Check sheet for the modelled part. Datum: model origin and axes. Units: mm. Round coordinates to 2 decimals unless told otherwise and drop trailing zeros. Loops run counter-clockwise (first coordinate to the right, second up) from the corner with the lowest first, then second, coordinate; pieces in that order, holes last. Notation, with made-up numbers: M -14,84 L 5,84 A13 cw 5,96 Z; hole C 11.5,-20.5 d2. An arc over 180 degrees is marked long. Write item = value, one per line. Start each with the question number.
(1) Cross-section at C-C on x = -23. Record the boundary of the cut face in (y, z), plus the area to 3 significant figures.
(2) Cross-section at D-D on z = 2.15. Record the boundary of the cut face in (x, y), plus the area to 3 significant figures.
(3) Go/stop test with flat-tipped pins: P1, Ø1, axis at x = 41.5, z = 2.5, coming from the +Y side; P2, Ø1, axis at x = -47.5, z = 2, coming from the +Y side. Record where each tip stops, or that it passes through.
(4) Cross-section at A-A on x = 0. Record the boundary of the cut face in (y, z), plus the area to 3 significant figures.
(5) Scan lines: L1, parallel to Y at x = 0, z = 2.95; L2, parallel to Y at x = 23, z = 1.25; L3, parallel to X at y = -12, z = 1.25. Record each from-to range of solid material in increasing order. Write a range as from..to.
(6) Mould release check, pull along Y, two halves, no side actions. Record for faces 1 (the face through (-1, -48.822, 2)), 2 (the face through (62, 14, 2)), 3 (the face through (-40.8, 41.8, 1.7)), 4 (the face through (0.89, 90.77, 1.69)): pulls with the +Y half, pulls with the -Y half, needs draft (parallel to the pull), parting line crosses it, or undercut.
(7) Cross-section at B-B on x = 15.5. Record the boundary of the cut face in (y, z), plus the area to 3 significant figures.
from build123d import *

# Parameters (mm, degrees)
SKETCH1_W           = 70
SKETCH1_H           = 105
BOSS_EXTRUDE1_DEPTH = 3
SKETCH2_R           = 17.5
CUT_EXTRUDE3_DEPTH  = 3
CUT_EXTRUDE6_DEPTH  = 10
SCALE1_SCALE        = 1.771428571
SKETCH6_R           = 30.999999993
CUT_EXTRUDE7_DEPTH  = 0.31
SKETCH7_W           = 123.99999997
SKETCH7_H           = 38.57142855
CUT_EXTRUDE8_DEPTH  = 10
SKETCH9_R           = 2.5
CUT_EXTRUDE9_DEPTH  = 5.004285713
SKETCH10_R          = 2.5
CUT_EXTRUDE10_DEPTH = 5.004285713


with BuildPart() as part:
    # Sketch1 → Boss-Extrude1 (new body)
    with BuildSketch(Plane.XY):
        Rectangle(SKETCH1_W, SKETCH1_H)
    extrude(amount=BOSS_EXTRUDE1_DEPTH)

    # Sketch2 → Cut-Extrude3 (cut)
    with BuildSketch(Plane(origin=(0, 0, 0), x_dir=(-1, 0, 0), z_dir=(0, 0, -1))):
        with Locations((0, 20.5)):
            Circle(SKETCH2_R)
    extrude(amount=-CUT_EXTRUDE3_DEPTH, mode=Mode.SUBTRACT)

    # Sketch5 → Cut-Extrude6 (cut)
    with BuildSketch(Plane.XY.offset(3)):
        with BuildLine():
            Line((-35, 40.793543502), (-35, 52.5))
            Line((-35, 52.5), (35, 52.5))
            Line((35, 52.5), (35, 40.793543502))
            ThreePointArc((35, 40.793543502), (0, 48.07644174), (-35, 40.793543502))
        make_face()
    extrude(amount=-CUT_EXTRUDE6_DEPTH, mode=Mode.SUBTRACT)


with BuildPart() as part_1:
    # Scale1: scaled about (0, -7.267874882, 1.5)
    add(part.part.scale(SCALE1_SCALE).moved(Location((0, 5.606646334, -1.157142856))))

    # Sketch6 → Cut-Extrude7 (cut)
    with BuildSketch(Plane(origin=(0, 0, -1.157142856), x_dir=(-1, 0, 0), z_dir=(0, 0, -1))):
        with BuildLine():
            Line((61.999999985, -87.393353643), (61.999999985, 77.869494806))
            ThreePointArc((61.999999985, 77.869494806), (0, 90.770628825), (-61.999999985, 77.869494806))
            Line((-61.999999985, 77.869494806), (-61.999999985, -87.393353643))
            Line((-61.999999985, -87.393353643), (61.999999985, -87.393353643))
        make_face()
        with Locations((0, 41.92093204)):
            Circle(SKETCH6_R, mode=Mode.SUBTRACT)
    extrude(amount=-CUT_EXTRUDE7_DEPTH, mode=Mode.SUBTRACT)

    # Sketch7 → Cut-Extrude8 (cut)
    with BuildSketch(Plane.XY.offset(4.157142857)):
        with Locations((0, -68.107639368)):
            Rectangle(SKETCH7_W, SKETCH7_H)
    extrude(amount=-CUT_EXTRUDE8_DEPTH, mode=Mode.SUBTRACT)

    # Sketch9 → Cut-Extrude9 (cut)
    with BuildSketch(Plane.XY.offset(4.157142857)):
        with Locations((23, -13.821925093)):
            Circle(SKETCH9_R)
        with Locations((-23, -13.821925093)):
            Circle(SKETCH9_R)
        with Locations((0, -38.821925093)):
            Circle(SKETCH9_R)
    extrude(amount=-CUT_EXTRUDE9_DEPTH, mode=Mode.SUBTRACT)

    # Sketch10 → Cut-Extrude10 (cut)
    with BuildSketch(Plane.XY.offset(4.157142857)):
        with Locations((-40.233402491, 44.236817184)):
            Circle(SKETCH10_R)
        with Locations((0, 82.22093204)):
            Circle(SKETCH10_R)
        with Locations((40.233400771, 44.236847056)):
            Circle(SKETCH10_R)
    extrude(amount=-CUT_EXTRUDE10_DEPTH, mode=Mode.SUBTRACT)


solid = part_1.part
Result:
q1.outline = M -48.82,-0.85 L -16.32,-0.85 L -16.32,4.16 L -48.82,4.16 Z; M -11.32,-0.85 L 21.14,-0.85 L 21.14,4.16 L -11.32,4.16 Z; M 62.71,-0.85 L 89.06,-0.85 L 89.06,4.16 L 62.71,4.16 Z
q1.area = 457 mm^2
q2.outline = M -62,-48.82 L 62,-48.82 L 62,77.87 A155.43 ccw -62,77.87 Z; hole C -40.23,44.24 d5; hole C 0,41.92 d62; hole C -23,-13.82 d5; hole C 0,-38.82 d5; hole C 0,82.22 d5; hole C 23,-13.82 d5; hole C 40.23,44.24 d5
q2.area = 13,600 mm^2
q3.P1 = 85.27
q3.P2 = 83.49
q4.outline = M -48.82,-0.85 L -41.32,-0.85 L -41.32,4.16 L -48.82,4.16 Z; M -36.32,-0.85 L 10.92,-0.85 L 10.92,4.16 L -36.32,4.16 Z; M 72.92,-0.85 L 79.72,-0.85 L 79.72,4.16 L 72.92,4.16 Z; M 84.72,-0.85 L 90.77,-0.85 L 90.77,4.16 L 84.72,4.16 Z
q4.area = 338 mm^2
q5.L1 = -48.82..-41.32, -36.32..10.92, 72.92..79.72, 84.72..90.77
q5.L2 = -48.82..-16.32, -11.32..21.14, 62.71..89.06
q5.L3 = -62..-24.71, -21.29..21.29, 24.71..62
q6.face_1 = pulls with the -Y half
q6.face_2 = needs draft
q6.face_3 = undercut
q6.face_4 = pulls with the +Y half
q7.outline = M -48.82,-0.85 L 15.07,-0.85 L 15.07,4.16 L -48.82,4.16 Z; M 68.77,-0.85 L 90,-0.85 L 90,4.16 L 68.77,4.16 Z
q7.area = 426 mm^2
